from build123d import *

# Parameters (mm, degrees)
SKETCH_1_W          = 20
SKETCH_1_H          = 10
SKETCH_1_W_2        = 16
SKETCH_1_H_2        = 6
EXTRUDE_1_DEPTH     = 77
SKETCH_2_R          = 1.5
CUT_EXTRUDE_1_DEPTH = 80.711981534
SKETCH_3_R          = 1.5
CUT_EXTRUDE_2_DEPTH = 79.287930104


with BuildPart() as part:
    # 草图1 → 凸台-拉伸1 (new, symmetric)
    with BuildSketch(Plane(origin=(0, 0, 0), x_dir=(1, 0, 0), z_dir=(0, 1, 0))):
        Rectangle(SKETCH_1_W, SKETCH_1_H)
        Rectangle(SKETCH_1_W_2, SKETCH_1_H_2, mode=Mode.SUBTRACT)
    extrude(amount=EXTRUDE_1_DEPTH, both=True)

    # 草图2 → 切除-拉伸1 (cut, through all)
    with BuildSketch(Plane(origin=(10, 0, 0), x_dir=(0, 0, -1), z_dir=(1, 0, 0))):
        with Locations((0, 52)):
            Circle(SKETCH_2_R)
        with Locations((0, 72)):
            Circle(SKETCH_2_R)
        with Locations((0, 62)):
            Circle(SKETCH_2_R)
        with Locations((0, -72)):
            Circle(SKETCH_2_R)
        with Locations((0, -62)):
            Circle(SKETCH_2_R)
        with Locations((0, -52)):
            Circle(SKETCH_2_R)
    extrude(amount=-CUT_EXTRUDE_1_DEPTH, mode=Mode.SUBTRACT)

    # 草图3 → 切除-拉伸2 (cut, through all)
    with BuildSketch(Plane(origin=(0, 0, -5), x_dir=(-1, 0, 0), z_dir=(0, 0, -1))):
        with Locations((5, -15)):
            Circle(SKETCH_3_R)
        with Locations((-5, -15)):
            Circle(SKETCH_3_R)
        with Locations((-5, -25)):
            Circle(SKETCH_3_R)
        with Locations((5, -25)):
            Circle(SKETCH_3_R)
        with Locations((-5, 25)):
            Circle(SKETCH_3_R)
        with Locations((5, 25)):
            Circle(SKETCH_3_R)
        with Locations((5, 15)):
            Circle(SKETCH_3_R)
        with Locations((-5, 15)):
            Circle(SKETCH_3_R)
    extrude(amount=-CUT_EXTRUDE_2_DEPTH, mode=Mode.SUBTRACT)


solid = part.part
Could you check a few things on this model? Use its own coordinates, in mm. A direction names the side the tool comes from. Coordinates: 2 decimals unless noted, no trailing zeros. Order: outer loops, then holes, each group sorted by start corner. A loop starts at its lowest first (then second) coordinate and runs counter-clockwise, first axis right, second up.
Q1. Suppose I cut it at A-A on x = 0. Please give me the cut outline in (y, z).
Q2. Suppose I cut it at C-C on y = 37.5. Please give me the cut outline in (x, z).
Q3. Please list where these lines run through material, in increasing order: L1, parallel to Y at x = -5, z = 3.55; L2, parallel to Z at x = 6, y = 22.5; L3, parallel to X at y = 48.5, z = -0.5.
Q4. Thinking about a two-plate mould opening in X: for faces 1 (the flat face through (0, 1, -3)), 2 (the flat face through (10, 1, 0)), 3 (the cylindrical face through (-8.986, 73.265, -0.806)), which applies, released by +X, released by -X, zero draft, split by the parting line, or undercut?
Q5. Suppose I cut it at D-D on y = -15. Please give me the cut outline in (x, z), and give its area (3 significant figures).
Q6. Which directions (+Z, -Z, +X, -X, +Y, -Y) give clear straight access to the entire face, cutting with the end or side of a thin tool? Please do faces 4 (the flat face through (0, 1, 3)), 5 (the cylindrical face through (-4.805, 26.487, 3.986)).
Q7. Suppose I cut it at B-B on y = 62. Please give me the cut outline in (x, z), and give its area (3 significant figures).
Q8. Will this pin go through, and if not, where does the flat tip stop? pin 1 (2.5 mm diameter, centred on y = -62, z = 0, fed in from +X).
Answer:
1. outline: (-77, -5) - (77, -5) - (77, -3) - (-77, -3) - close; (-77, 3) - (77, 3) - (77, 5) - (-77, 5) - close
2. outline: (-10, -5) - (10, -5) - (10, 5) - (-10, 5) - close; hole (-8, -3) - (8, -3) - (8, 3) - (-8, 3) - close
3. L1: y = -77 to -26.5, -23.5 to -16.5, -13.5 to 13.5, 16.5 to 23.5, 26.5 to 77
3. L2: z = -5 to -3, 3 to 5
3. L3: x = -10 to -8, 8 to 10
4. face 1: undercut
4. face 2: released by +X
4. face 3: zero draft
5. outline: (-10, -5) - (-6.5, -5) - (-6.5, -3) - (-8, -3) - (-8, 3) - (-6.5, 3) - (-6.5, 5) - (-10, 5) - close; (-3.5, -5) - (3.5, -5) - (3.5, -3) - (-3.5, -3) - close; (-3.5, 3) - (3.5, 3) - (3.5, 5) - (-3.5, 5) - close; (6.5, -5) - (10, -5) - (10, 5) - (6.5, 5) - (6.5, 3) - (8, 3) - (8, -3) - (6.5, -3) - close
5. area: 80.0 mm2
6. face 4: +Y, -Y
6. face 5: +Z, -Z
7. outline: (-10, -5) - (10, -5) - (10, -1.5) - (8, -1.5) - (8, -3) - (-8, -3) - (-8, -1.5) - (-10, -1.5) - close; (-10, 1.5) - (-8, 1.5) - (-8, 3) - (8, 3) - (8, 1.5) - (10, 1.5) - (10, 5) - (-10, 5) - close
7. area: 92.0 mm2
8. pin 1: passes through
